For this review, take the finished solid that the model builds, in its own axes (mm). A direction names the side the tool comes from. Round coordinates to 2 decimals unless told otherwise and drop trailing zeros. Write each loop counter-clockwise with the first axis right and the second up, starting at its lowest first coordinate (ties: lowest second). Pieces come first, ordered by that corner, then holes. Notation, with made-up numbers: (-9.5, 51) -> (18.5, 51) arc R5 ccw to (18.5, 55) -> close; hole circle Ø1 at (11.25, 75). An arc over 180 degrees is marked (long way). Write each question's results on one line, items separated by ' | '. Start each with the question number.
Item 1: Add section A-A (y = 8). State the section outline as (x, z) points, plus the area to 3 significant figures.
Item 2: Add section D-D (y = 18). State the section outline as (x, z) points, plus the area to 3 significant figures.
Item 3: Add section C-C (z = 29). State the section outline as (x, y) points, plus the area to 3 significant figures.
Item 4: Tool access review of faces 1 (the flat face through (0, 2.5, -6)), 2 (the cylindrical face through (7.15, -6.99, 45.04)), 3 (the cylindrical face through (-7.15, 0.04, -16.99)), 4 (the flat face through (0, 5, 20)), 5 (the flat face through (0, 25, 30)): name each direction out of +Z, -Z, +X, -X, +Y, -Y from which nothing blocks a thin tool from reaching the whole face with its end or side.
Item 5: To check wall thickness, follow line 1 along X through (y, z) = (-0.2, -10); line 2 along Y through (x, z) = (0, 44.25); line 3 along Z through (x, y) = (0, 6.5). State the ranges of each line that lie inside material, in increasing order.
Item 6: Clearance check with flat-ended pins moving along their axes: pin 1 (8 mm diameter, centred on x = 0.5, z = 35, fed in from -Y); pin 2 (10 mm diameter, centred on x = 0.5, y = -4, fed in from +Z); pin 3 (2.5 mm diameter, centred on x = -4, z = 11.5, fed in from -Y); pin 4 (12 mm diameter, centred on y = 16, z = 3, fed in from -X). State where each tip first meets the part, or that it passes through.
Item 7: Add section B-B (x = 1). State the section outline as (y, z) points.
Item 8: The part is to be moulded in two halves that separate along Z. For faces 6 (the flat face through (0, 4, 47.5)), 7 (the flat face through (0, 12, 22)), 8 (the flat face through (0, -4, 9)), say which applies: +Z half, -Z half, draft (parallel to the pull), parting line (faces both ways), or undercut.
from build123d import *

# Parameters (mm, degrees)
SKETCH1_W               = 20
SKETCH1_H               = 10
BOSS_EXTRUDE1_DEPTH     = 10
SKETCH3_W               = 20
SKETCH3_H               = 5
BOSS_EXTRUDE2_DEPTH     = 20
FILLET1_R               = 10
BOSS_EXTRUDE3_DEPTH     = 20
CUT_EXTRUDE1_DEPTH      = 56.733742024
CUT_EXTRUDE1_DEPTH_BACK = 56.733742024
SKETCH5_R               = 2.75
CHAMFER1_SIZE           = 10
SKETCH6_W               = 20
SKETCH6_H               = 5
BOSS_EXTRUDE4_DEPTH     = 20
FILLET2_R               = 10
CUT_EXTRUDE2_DEPTH      = 73.672209269
CUT_EXTRUDE2_DEPTH_BACK = 5
SKETCH7_R               = 2.75
CHAMFER2_SIZE           = 5
CHAMFER3_SIZE           = 5


# Some blends are built 0.0001 mm under size
with BuildPart() as part:
    # Sketch1 → Boss-Extrude1 (new body)
    with BuildSketch(Plane.XY):
        Rectangle(SKETCH1_W, SKETCH1_H)
    extrude(amount=BOSS_EXTRUDE1_DEPTH)

    # Sketch3 → Boss-Extrude2 (add)
    with BuildSketch(Plane(origin=(0, 0, 0), x_dir=(-1, 0, 0), z_dir=(0, 0, -1))):
        Rectangle(SKETCH3_W, SKETCH3_H)
    extrude(amount=BOSS_EXTRUDE2_DEPTH)

    # Fillet1
    fillet1_edges = [part.edges().sort_by_distance(p)[0] for p in [
        (-10, 0, -20),
        (10, 0, -20),
    ]]
    fillet(fillet1_edges, radius=FILLET1_R - 0.0001)  # a hair under: the kernel refuses the full size

    # Sketch4 → Boss-Extrude3 (add)
    with BuildSketch(Plane.ZY.offset(10)):
        Polygon((20, -5), (20, 15), (40, 15), (40, 10), (50, 10), (50, 25), (10, 25), (10, -5), align=None)
    extrude(amount=-BOSS_EXTRUDE3_DEPTH)

    # Sketch5 → Cut-Extrude1 (cut, two sides: drawn at the far end of the back side and taken through both)
    with BuildSketch(Plane(origin=(0, 2.5, 0), x_dir=(1, 0, 0), z_dir=(0, 1, 0)).offset(-CUT_EXTRUDE1_DEPTH_BACK)):
        with Locations(Location((0, 10, 0), (0, 0, 270))):
            Circle(SKETCH5_R)
    extrude(amount=CUT_EXTRUDE1_DEPTH + CUT_EXTRUDE1_DEPTH_BACK, mode=Mode.SUBTRACT)

    # Chamfer1
    # the kernel refuses this chamfer: 10 mm, written as the material it takes off along each edge
    with BuildSketch(Plane(origin=(35.71682988, 5, 0), x_dir=(0, -0.9996219169112968, -0.027495876610586372), z_dir=(-1, 0, 0))) as chamfer1_piece_1_section:
        Polygon((CHAMFER1_SIZE * 0.999621916911, CHAMFER1_SIZE * 0.0274958766106), (-CHAMFER1_SIZE * 0.0274958766106, CHAMFER1_SIZE * 0.999621916911), (0, 0), align=None)
    chamfer1_piece_1 = extrude(amount=71.433659759, mode=Mode.PRIVATE)
    chamfer1_piece_1 = split(chamfer1_piece_1, bisect_by=Plane(origin=(0, -2.5, 0.578931494), z_dir=(0, -1, 0)), keep=Keep.TOP, mode=Mode.PRIVATE)
    add(chamfer1_piece_1, mode=Mode.SUBTRACT)
    with BuildSketch(Plane(origin=(35.71682988, 5, 0), x_dir=(0, -0.9996219169112968, -0.027495876610586372), z_dir=(-1, 0, 0))) as chamfer1_piece_2_section:
        Polygon((CHAMFER1_SIZE * 0.999621916911, CHAMFER1_SIZE * 0.0274958766106), (-CHAMFER1_SIZE * 0.0274958766106, CHAMFER1_SIZE * 0.999621916911), (0, 0), align=None)
    chamfer1_piece_2 = extrude(amount=71.433659759, mode=Mode.PRIVATE)
    chamfer1_piece_2 = split(chamfer1_piece_2, bisect_by=Plane(origin=(0, 2.5, 4.466280687), z_dir=(0, 1, 0)), keep=Keep.TOP, mode=Mode.PRIVATE)
    chamfer1_piece_2 = split(chamfer1_piece_2, bisect_by=Plane(origin=(0, 3.939233337, 10), z_dir=(0, 0, -1)), keep=Keep.TOP, mode=Mode.PRIVATE)
    add(chamfer1_piece_2, mode=Mode.SUBTRACT)
    with BuildSketch(Plane(origin=(-35.71682988, -5, 0), x_dir=(0, -0.027495876610586403, 0.9996219169112968), z_dir=(1, 0, 0))) as chamfer1_piece_3_section:
        Polygon((CHAMFER1_SIZE * 0.999621916911, -CHAMFER1_SIZE * 0.0274958766106), (-CHAMFER1_SIZE * 0.0274958766106, -CHAMFER1_SIZE * 0.999621916911), (0, 0), align=None)
    chamfer1_piece_3 = extrude(amount=71.433659759, mode=Mode.PRIVATE)
    chamfer1_piece_3 = split(chamfer1_piece_3, bisect_by=Plane(origin=(0, -2.5, 4.487529346), z_dir=(0, -1, 0)), keep=Keep.TOP, mode=Mode.PRIVATE)
    add(chamfer1_piece_3, mode=Mode.SUBTRACT)
    with BuildSketch(Plane(origin=(-35.71682988, -5, 0), x_dir=(0, -0.027495876610586403, 0.9996219169112968), z_dir=(1, 0, 0))) as chamfer1_piece_4_section:
        Polygon((CHAMFER1_SIZE * 0.999621916911, -CHAMFER1_SIZE * 0.0274958766106), (-CHAMFER1_SIZE * 0.0274958766106, -CHAMFER1_SIZE * 0.999621916911), (0, 0), align=None)
    chamfer1_piece_4 = extrude(amount=71.433659759, mode=Mode.PRIVATE)
    chamfer1_piece_4 = split(chamfer1_piece_4, bisect_by=Plane(origin=(0, 2.5, 0.578931494), z_dir=(0, 1, 0)), keep=Keep.TOP, mode=Mode.PRIVATE)
    add(chamfer1_piece_4, mode=Mode.SUBTRACT)

    # Sketch6 → Boss-Extrude4 (add)
    with BuildSketch(Plane.XZ.offset(-10)):
        with Locations((0, 45)):
            Rectangle(SKETCH6_W, SKETCH6_H)
    extrude(amount=BOSS_EXTRUDE4_DEPTH)

    # Fillet2
    fillet2_edges = [part.edges().sort_by_distance(p)[0] for p in [
        (10, -10, 45),
        (-10, -10, 45),
    ]]
    fillet(fillet2_edges, radius=FILLET2_R - 0.0001)  # a hair under: the kernel refuses the full size

    # Sketch7 → Cut-Extrude2 (cut, two sides: drawn at the far end of the back side and taken through both)
    with BuildSketch(Plane.XY.offset(47.5).offset(-CUT_EXTRUDE2_DEPTH_BACK)):
        Circle(SKETCH7_R)
    extrude(amount=CUT_EXTRUDE2_DEPTH + CUT_EXTRUDE2_DEPTH_BACK, mode=Mode.SUBTRACT)

    # Chamfer2
    # the kernel refuses this chamfer: 5 mm, written as the material it takes off along each edge
    with BuildSketch(Plane(origin=(-22.85841494, 10, 40), x_dir=(0, -0.027495876610586317, 0.9996219169112968), z_dir=(1, 0, 0))) as chamfer2_piece_1_section:
        Polygon((CHAMFER2_SIZE * 0.999621916911, -CHAMFER2_SIZE * 0.0274958766106), (-CHAMFER2_SIZE * 0.0274958766106, -CHAMFER2_SIZE * 0.999621916911), (0, 0), align=None)
    chamfer2_piece_1 = extrude(amount=45.71682988, mode=Mode.PRIVATE)
    chamfer2_piece_1 = split(chamfer2_piece_1, bisect_by=Plane(origin=(0, 11.959930185, 42.5), z_dir=(0, 0, -1)), keep=Keep.TOP, mode=Mode.PRIVATE)
    chamfer2_piece_1 = split(chamfer2_piece_1, bisect_by=Plane(origin=(0, 15, 41.043890797), z_dir=(0, -1, 0)), keep=Keep.TOP, mode=Mode.PRIVATE)
    add(chamfer2_piece_1, mode=Mode.SUBTRACT)
    with BuildSketch(Plane(origin=(-22.85841494, 10, 50), x_dir=(0, -0.027495876610586317, -0.9996219169112968), z_dir=(1, 0, 0))) as chamfer2_piece_2_section:
        Polygon((CHAMFER2_SIZE * 0.999621916911, CHAMFER2_SIZE * 0.0274958766106), (-CHAMFER2_SIZE * 0.0274958766106, CHAMFER2_SIZE * 0.999621916911), (0, 0), align=None)
    chamfer2_piece_2 = extrude(amount=45.71682988, mode=Mode.PRIVATE)
    chamfer2_piece_2 = split(chamfer2_piece_2, bisect_by=Plane(origin=(0, 11.967005421, 47.5), z_dir=(0, 0, 1)), keep=Keep.TOP, mode=Mode.PRIVATE)
    add(chamfer2_piece_2, mode=Mode.SUBTRACT)

    # Chamfer3
    chamfer3_edges = [part.edges().sort_by_distance(p)[0] for p in [
        (0, 25, 10),
        (0, 25, 50),
        (0, 15, 20),
        (0, -5, 20),
    ]]
    chamfer(chamfer3_edges, length=CHAMFER3_SIZE)


solid = part.part
Responses:
1) outline: (-10, 10) -> (10, 10) -> (10, 20) -> (-10, 20) -> close; (-10, 42.5) -> (10, 42.5) -> (10, 47.5) -> (-10, 47.5) -> close | area: 300 mm^2
2) outline: (-10, 10) -> (10, 10) -> (10, 50) -> (-10, 50) -> close | area: 800 mm^2
3) outline: (-10, 15) -> (10, 15) -> (10, 25) -> (-10, 25) -> close | area: 200 mm^2
4) face 1: -Z, +X, -X, +Y | face 2: +Z, +X, -Y | face 3: -Z, -X, +Y, -Y | face 4: +X, -X, -Y | face 5: +Z, -Z, +X, -X, +Y
5) line 1: x = -10 to -2.75, 2.75 to 10 | line 2: y = -10 to -2.75, 2.75 to 25 | line 3: z = 10 to 20, 42.5 to 47.5
6) pin 1: stops at y = 15 | pin 2: stops at z = 47.5 | pin 3: stops at y = -5 | pin 4: passes through
7) outline: (-9.95, 42.5) -> (-2.56, 42.5) -> (-2.56, 47.5) -> (-9.95, 47.5) -> close; (-5, 10) -> (-2.5, 7.5) -> (-2.5, -7.44) -> (2.5, -7.44) -> (2.5, 7.5) -> (5, 10) -> (20, 10) -> (25, 15) -> (25, 45) -> (20, 50) -> (15, 50) -> (12.5, 47.5) -> (2.56, 47.5) -> (2.56, 42.5) -> (12.5, 42.5) -> (15, 40) -> (15, 25) -> (10, 20) -> (0, 20) -> (-5, 15) -> close; (-2.5, -19.95) -> (2.5, -19.95) -> (2.5, -12.56) -> (-2.5, -12.56) -> close
8) face 6: +Z half | face 7: undercut | face 8: -Z half
